```python
from build123d import *

# Parameters (mm, degrees)
SKETCH1_W           = 25.4
SKETCH1_H           = 83.82
BOSS_EXTRUDE1_DEPTH = 3.175
SKETCH2_R           = 2.4892
CUT_EXTRUDE1_DEPTH  = 88.641502868
FILLET1_R           = 6.35


with BuildPart() as part:
    # Sketch1 → Boss-Extrude1 (new body)
    with BuildSketch(Plane.XY):
        with Locations((12.7, 41.91)):
            Rectangle(SKETCH1_W, SKETCH1_H)
    extrude(amount=BOSS_EXTRUDE1_DEPTH)

    # Sketch2 → Cut-Extrude1 (cut, through all)
    with BuildSketch(Plane.XY.offset(3.175)):
        with Locations((12.7, 12.7)):
            Circle(SKETCH2_R)
        with Locations((12.7, 38.1)):
            Circle(SKETCH2_R)
        with Locations((12.7, 63.5)):
            Circle(SKETCH2_R)
    extrude(amount=-CUT_EXTRUDE1_DEPTH, mode=Mode.SUBTRACT)

    # Fillet1
    fillet1_edges = [part.edges().sort_by_distance(p)[0] for p in [
        (0, 83.82, 1.5875),
        (25.4, 83.82, 1.5875),
        (25.4, 0, 1.5875),
        (0, 0, 1.5875),
    ]]
    fillet(fillet1_edges, radius=FILLET1_R)


solid = part.part
```
Input: part model. Units: mm. Frame: model coordinates. Coordinates: 2 decimals unless noted, no trailing zeros. Write each loop counter-clockwise with the first axis right and the second up, starting at its lowest first coordinate (ties: lowest second). Pieces come first, ordered by that corner, then holes.
1) Section C-C on x = 12.7. Output: boundary loops of the cut face in (y, z) (3 decimals), and give its area (3 significant figures).
2) Material intervals for line 1 along Y through (x, z) = (12.7, 1.9); line 2 along X through (y, z) = (10.5, 1.9); line 3 along Y through (x, z) = (14.5, 0.5), sorted ascending.
3) Section A-A on z = 1.25. Output: boundary loops of the cut face in (x, y), and give its area (3 significant figures).
4) Mould query, pull axis X, two halves, no side actions, for faces 1 (the cylindrical face through (12.38, 15.17, 1.61)), 2 (the cylindrical face through (23.5, 82, 1.6)), 3 (the flat face through (0, 41, 2)). Classes: pulls with the +X half, pulls with the -X half, needs draft (parallel to the pull), parting line crosses it, or undercut.
5) Pin query (flat end, axial travel): pin 1 Ø4.5 at (x, y) = (12.7, 38.1) entering from +Z. Return the tip coordinate at first contact, or that it passes through.
6) Section B-B on y = 38.1. Output: boundary loops of the cut face in (x, z) (3 decimals).
7) Section D-D on x = 22. Output: boundary loops of the cut face in (y, z) (3 decimals), and give its area (3 significant figures).
Check result:
1. outline: (0, 0) - (10.211, 0) - (10.211, 3.175) - (0, 3.175) - close; (15.189, 0) - (35.611, 0) - (35.611, 3.175) - (15.189, 3.175) - close; (40.589, 0) - (61.011, 0) - (61.011, 3.175) - (40.589, 3.175) - close; (65.989, 0) - (83.82, 0) - (83.82, 3.175) - (65.989, 3.175) - close
1. area: 219 mm2
2. line 1: y = 0 to 10.21, 15.19 to 35.61, 40.59 to 61.01, 65.99 to 83.82
2. line 2: x = 0 to 11.54, 13.86 to 25.4
2. line 3: y = 0 to 10.98, 14.42 to 36.38, 39.82 to 61.78, 65.22 to 83.82
3. outline: (0, 6.35) arc R6.35 ccw to (6.35, 0) - (19.05, 0) arc R6.35 ccw to (25.4, 6.35) - (25.4, 77.47) arc R6.35 ccw to (19.05, 83.82) - (6.35, 83.82) arc R6.35 ccw to (0, 77.47) - close; hole circle Ø4.98 at (12.7, 12.7); hole circle Ø4.98 at (12.7, 38.1); hole circle Ø4.98 at (12.7, 63.5)
3. area: 2,040 mm2
4. face 1: undercut
4. face 2: pulls with the +X half
4. face 3: pulls with the -X half
5. pin 1: passes through
6. outline: (0, 0) - (10.211, 0) - (10.211, 3.175) - (0, 3.175) - close; (15.189, 0) - (25.4, 0) - (25.4, 3.175) - (15.189, 3.175) - close
7. outline: (0.727, 0) - (83.093, 0) - (83.093, 3.175) - (0.727, 3.175) - close
7. area: 262 mm2
